Read the model definition and answer for the solid it produces. Units are mm, in the model's axes. Face numbers are marked on the shaded views. A direction names the side the tool comes from. Give positions to 0.01 mm unless a question says otherwise; leave off trailing zeros. Write each loop counter-clockwise with the first axis right and the second up, starting at its lowest first coordinate (ties: lowest second). Pieces come first, ordered by that corner, then holes. Notation, with made-up numbers: M -30.75,3 L -8.75,3 A31 ccw -8.75,28 Z; hole C 23.25,58 d7. An arc over 180 degrees is marked long. Use a Markdown table: item, result. Add a question column.
Item 1: Consider probe 1 along X at (y, z) = (72.5, 0.5); probe 2 along X at (y, z) = (64.5, 1); probe 3 along Y at (x, z) = (-112, 1.75). Determine where each line is inside the solid, lowest interval first. Write a range as [from, to].
Item 2: A cutting plane is placed at A-A on z = -0.5. Determine the outline of the cut face in (x, y).
Item 3: The mould has two halves that part along X. Classify the marked faces 3, 4 and 5: pulls with the +X half, pulls with the -X half, needs draft (parallel to the pull), parting line crosses it, or undercut.
Item 4: A cutting plane is placed at D-D on x = -87.5. Determine the outline of the cut face in (y, z), then the cut area to 3 significant figures.
Item 5: A cutting plane is placed at C-C on y = 64.5. Determine the outline of the cut face in (x, z), then the cut area to 3 significant figures.
Item 6: For the marked faces 1 and 2, determine the directions among +Z, -Z, +X, -X, +Y, -Y from which every point of the face is accessible in a straight line to the end or side of a thin tool.
Item 7: Given P1, Ø1, axis at x = -89.5, z = 0, coming from the +Y side; P2, Ø2.5, axis at x = -103.15, y = 72.5, coming from the -Z side, each flat-ended and moving along its own axis, determine where each tip first touches the part or whether it passes through.
Item 8: A cutting plane is placed at B-B on y = 72.5. Determine the outline of the cut face in (x, z).
from build123d import *

# Parameters (mm, degrees)
EXTRUDE_1_DEPTH     = 3.5
SKETCH_3_R          = 1.6
CUT_EXTRUDE_1_DEPTH = 16
CUT_EXTRUDE_2_DEPTH = 13
FILLET_1_R          = 1
FILLET_2_R          = 3
FILLET_3_R          = 4


with BuildPart() as part:
    # 草图2 → 凸台-拉伸1 (new, symmetric)
    with BuildSketch(Plane.XY):
        with BuildLine():
            Line((-117.154590294, 76.5), (-117.154590294, 66.5))
            ThreePointArc((-117.154590294, 66.5), (-111.882512356, 53.772077939), (-99.154590294, 48.5))
            Line((-99.154590294, 48.5), (-82.154590294, 48.5))
            Line((-82.154590294, 48.5), (-82.154590294, 53))
            Line((-82.154590294, 53), (-99.154590294, 53))
            Line((-99.154590294, 53), (-99.154590294, 76.5))
            Line((-99.154590294, 76.5), (-117.154590294, 76.5))
        make_face()
    extrude(amount=EXTRUDE_1_DEPTH, both=True)

    # 草图3 → 切除-拉伸1 (cut)
    with BuildSketch(Plane.XY.offset(3.5)):
        with Locations((-103.154590294, 72.5)):
            Circle(SKETCH_3_R)
        with Locations((-111.154590294, 72.5)):
            Circle(SKETCH_3_R)
        with Locations((-111.154590294, 64.5)):
            Circle(SKETCH_3_R)
        with Locations((-103.154590294, 64.5)):
            Circle(SKETCH_3_R)
    extrude(amount=-CUT_EXTRUDE_1_DEPTH, mode=Mode.SUBTRACT)

    # 草图4 → 切除-拉伸2 (cut)
    with BuildSketch(Plane.XY.offset(3.5)):
        with BuildLine():
            Line((-90.683951349, 48.5), (-90.683951349, 46.627419574))
            Line((-90.683951349, 46.627419574), (-65.683951349, 46.627419574))
            Line((-65.683951349, 46.627419574), (-65.683951349, 73.5))
            ThreePointArc((-65.683951349, 73.5), (-73.006281819, 55.82233047), (-90.683951349, 48.5))
        make_face()
    extrude(amount=-CUT_EXTRUDE_2_DEPTH, mode=Mode.SUBTRACT)

    # 圆角1
    fillet_1_edges = [part.edges().sort_by_distance(p)[0] for p in [
        (-82.154590294, 53, 0),
        (-82.154590294, 50, 0),
    ]]
    fillet(fillet_1_edges, radius=FILLET_1_R)

    # 圆角2
    fillet_2_edges = [part.edges().sort_by_distance(p)[0] for p in [
        (-117.154590294, 76.5, 0),
        (-99.154590294, 76.5, 0),
    ]]
    fillet(fillet_2_edges, radius=FILLET_2_R)

    # 圆角3
    fillet_3_edges = [part.edges().sort_by_distance(p)[0] for p in [
        (-99.154590294, 53, 0),
    ]]
    fillet(fillet_3_edges, radius=FILLET_3_R)


solid = part.part
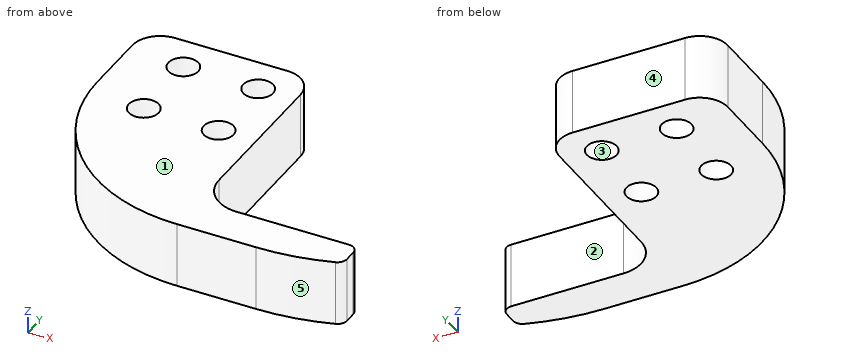
Filled in:
| question | item | result |
|---|---|---|
| 1 | probe 1 | [-117.15, -112.75], [-109.55, -104.75], [-101.55, -99.15] |
| 1 | probe 2 | [-117.04, -112.75], [-109.55, -104.75], [-101.55, -99.15] |
| 1 | probe 3 | [53.89, 63.14], [65.86, 71.14], [73.86, 76.5] |
| 2 | outline | M -117.15,66.5 A18 ccw -99.15,48.5 L -90.68,48.5 A25 ccw -82.84,49.76 A1 ccw -82.15,50.71 L -82.15,52 A1 ccw -83.15,53 L -95.15,53 A4 cw -99.15,57 L -99.15,73.5 A3 ccw -102.15,76.5 L -114.15,76.5 A3 ccw -117.15,73.5 Z; hole C -111.15,64.5 d3.2; hole C -111.15,72.5 d3.2; hole C -103.15,64.5 d3.2; hole C -103.15,72.5 d3.2 |
| 3 | face 3 | undercut |
| 3 | face 4 | needs draft |
| 3 | face 5 | pulls with the +X half |
| 4 | outline | M 48.7,-3.5 L 53,-3.5 L 53,3.5 L 48.7,3.5 Z |
| 4 | area | 30.1 mm² |
| 5 | outline | M -117.04,-3.5 L -112.75,-3.5 L -112.75,3.5 L -117.04,3.5 Z; M -109.55,-3.5 L -104.75,-3.5 L -104.75,3.5 L -109.55,3.5 Z; M -101.55,-3.5 L -99.15,-3.5 L -99.15,3.5 L -101.55,3.5 Z |
| 5 | area | 80.4 mm² |
| 6 | face 1 | +Z, +X, -X, +Y, -Y |
| 6 | face 2 | +Z, -Z, +X, +Y |
| 7 | P1 | y = 53 |
| 7 | P2 | through |
| 8 | outline | M -117.15,-3.5 L -112.75,-3.5 L -112.75,3.5 L -117.15,3.5 Z; M -109.55,-3.5 L -104.75,-3.5 L -104.75,3.5 L -109.55,3.5 Z; M -101.55,-3.5 L -99.15,-3.5 L -99.15,3.5 L -101.55,3.5 Z |
